Geometry check sheet. Reference: the model listing, model coordinates, mm. A direction names the side the tool comes from. Give positions to 0.01 mm unless a question says otherwise; leave off trailing zeros. Write each loop counter-clockwise with the first axis right and the second up, starting at its lowest first coordinate (ties: lowest second). Pieces come first, ordered by that corner, then holes. Notation, with made-up numbers: (21.25, 46) - (74.25, 46) arc R35 cw to (74.25, 80) - close; hole circle Ø9 at (43.5, 38). An arc over 180 degrees is marked (long way). Write item = value, one per line. Start each with the question number.
(1) Draft check along X on faces 1 (the flat face through (3, 0, -1)), 2 (the cylindrical face through (-6.094, -1.035, 0.268)), 3 (the cylindrical face through (-0.99, -1.24, -4.44)). Enter one of: pulls with the +X half, pulls with the -X half, needs draft (parallel to the pull), parting line crosses it, or undercut.
(2) Depth check by flat-ended pin: pin 1 Ø5.5 at (x, z) = (0, -1) entering from -Y. Enter the tip coordinate at first touch or a pass-through.
(3) Section check C-C, the plane y = -1.1. Enter the section's corners in (x, z), plus the area to 3 significant figures.
(4) Access from +Z, -Z, +X, -X, +Y, -Y to the whole of each face (thin tool, end or side, straight path). Record for faces 4 (the cylindrical face through (-0.596, -0.304, -2.685)), 5 (the flat face through (0, -0.6, -3)).
(5) Section check B-B, the plane z = -0.25. Enter the section's corners in (x, y).
(6) Section check A-A, the plane x = 0. Enter the section's corners in (y, z).
(7) Thickness scan on L1, parallel to Z at x = 0, y = -2; L2, parallel to Z at x = 0, y = -0.9; L3, parallel to Y at x = -4.25, z = 1. Record the ranges inside material, lowest first.
(8) Section check D-D, the plane z = -5. Enter the section's corners in (x, y).
```python
from build123d import *

# Parameters (mm, degrees)
F0_R     = 6.1
F1_DEPTH = 0.6
F2_R     = 6.1
F2_R_2   = 4.55
F3_DEPTH = 1.3
F4_R     = 2.75
F5_DEPTH = 0.6
F6_R     = 6.1
F6_R_2   = 5.7
F7_DEPTH = 0.2


with BuildPart() as f1:
    # F0 (on Front) → F1 (new body)
    with BuildSketch(Plane.XZ):
        Circle(F0_R)
    extrude(amount=F1_DEPTH)

    # F2 (on face) → F3 (join)
    with BuildSketch(Plane.XZ.offset(0.6)):
        Circle(F2_R)
        Circle(F2_R_2, mode=Mode.SUBTRACT)
    extrude(amount=F3_DEPTH)

    # F4 (on face) → F5 (cut)
    with BuildSketch(Plane.XZ.offset(0.6)):
        Circle(F4_R)
    extrude(amount=-F5_DEPTH, mode=Mode.SUBTRACT)

    # F6 (on face) → F7 (join)
    with BuildSketch(Plane.XZ.offset(1.9)):
        Circle(F6_R)
        Circle(F6_R_2, mode=Mode.SUBTRACT)
    extrude(amount=F7_DEPTH)


solid = f1.part
```
Model answer:
q1.face_1 = needs draft
q1.face_2 = parting line crosses it
q1.face_3 = undercut
q2.pin_1 = -0.6
q3.outline = circle Ø12.2 at (0, 0); hole circle Ø9.1 at (0, 0)
q3.area = 51.9 mm²
q4.face_4 = +Y, -Y
q4.face_5 = -Y
q5.outline = (-6.09, -2.1) - (-5.69, -2.1) - (-5.69, -1.9) - (-4.54, -1.9) - (-4.54, -0.6) - (-2.74, -0.6) - (-2.74, 0) - (-6.09, 0) - close; (2.74, -0.6) - (4.54, -0.6) - (4.54, -1.9) - (5.69, -1.9) - (5.69, -2.1) - (6.09, -2.1) - (6.09, 0) - (2.74, 0) - close
q6.outline = (-2.1, -6.1) - (0, -6.1) - (0, -2.75) - (-0.6, -2.75) - (-0.6, -4.55) - (-1.9, -4.55) - (-1.9, -5.7) - (-2.1, -5.7) - close; (-2.1, 5.7) - (-1.9, 5.7) - (-1.9, 4.55) - (-0.6, 4.55) - (-0.6, 2.75) - (0, 2.75) - (0, 6.1) - (-2.1, 6.1) - close
q7.L1 = -6.1 to -5.7, 5.7 to 6.1
q7.L2 = -6.1 to -4.55, 4.55 to 6.1
q7.L3 = -0.6 to 0
q8.outline = (-3.49, -2.1) - (-2.74, -2.1) - (-2.74, -1.9) - (2.74, -1.9) - (2.74, -2.1) - (3.49, -2.1) - (3.49, 0) - (-3.49, 0) - close
